For this review, use the dimensioned drawing (mm, ordinates from the lowest corner) and the shaded views. A direction names the side the tool comes from. Coordinates: 2 decimals unless noted, no trailing zeros. Loops run counter-clockwise (first coordinate to the right, second up) from the corner with the lowest first, then second, coordinate; pieces in that order, holes last. Notation, with made-up numbers: M 44.25,36.25 L 60.25,36.25 A23 ccw 60.25,64.25 Z; hole C 27.5,-7 d7. An arc over 180 degrees is marked long. Write item = value, one per line. Start each with the question number.
Q1. We need section B-B on x = 56. Give the boundary of the cut face in (y, z).
Q2. Wall thickness on probe 1 along X at (y, z) = (49.5, 6) (1 decimal); probe 2 along Y at (x, z) = (50, 29); probe 3 along X at (y, z) = (69, 44): over which ranges is each line inside the solid? List them lowest first.
Q3. We need section C-C on x = 30.5. Give the boundary of the cut face in (y, z) (1 decimal), and give its area (3 significant figures).
Q4. Mouldability with a two-part tool opening along Y and no side actions: class the marked faces 3, 4 and 5 as released by +Y, released by -Y, zero draft, split by the parting line, or undercut.
Q5. We need section A-A on z = 25. Give the boundary of the cut face in (x, y), and give its area (3 significant figures).
Q6. For the marked faces 1 and 2, list the 3-axis set-ups (+Z, -Z, +X, -X, +Y, -Y) from which the entire face can be reached by the end or side of a thin tool; tool diameter is ignored.
Q7. Clearance check with flat-ended pins moving along their axes: pin 1 Ø3 at (y, z) = (89.5, 21) entering from -X (1 decimal); pin 2 Ø2 at (x, z) = (86.5, 15) entering from -Y; pin 3 Ø4 at (x, y) = (217, 30.5) entering from +Z. State where each tip first meets the part, or that it passes through.
Q8. We need section D-D on z = 14. Give the boundary of the cut face in (x, y).
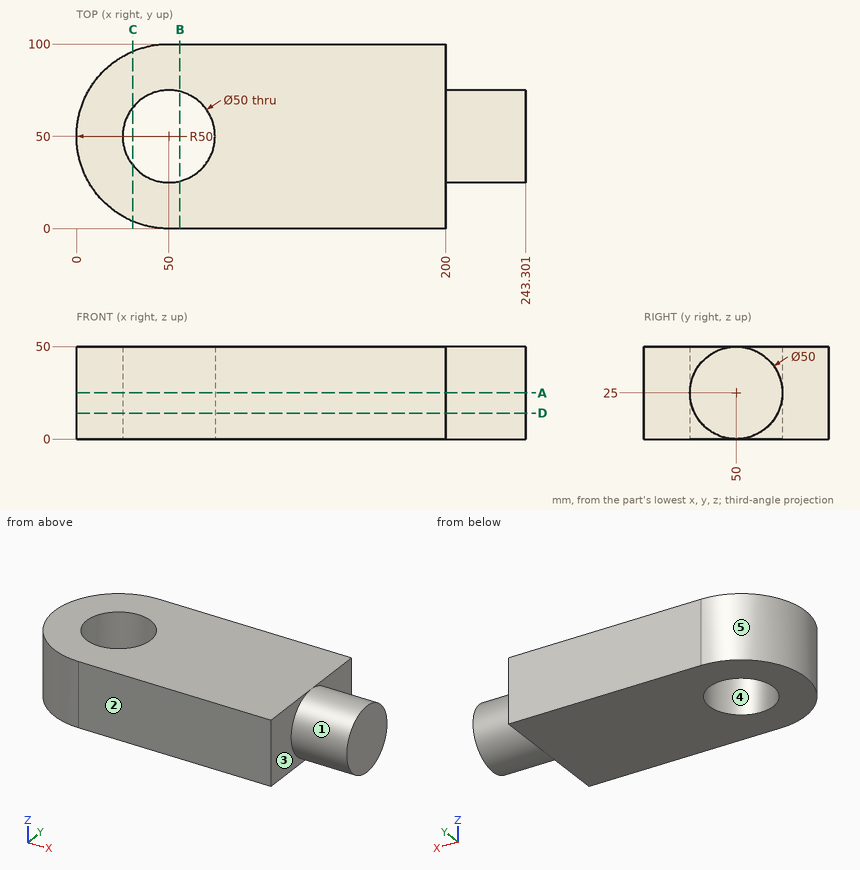
Returned:
q1.outline = M 0,0 L 25.73,0 L 25.73,50 L 0,50 Z; M 74.27,0 L 100,0 L 100,50 L 74.27,50 Z
q2.probe_1 = 0 to 25, 75 to 243.3
q2.probe_2 = 0 to 25, 75 to 100
q2.probe_3 = 3.75 to 33.75, 66.25 to 200
q3.outline = M 4,0 L 34.4,0 L 34.4,50 L 4,50 Z; M 65.6,0 L 96,0 L 96,50 L 65.6,50 Z
q3.area = 3,040 mm^2
q4.face_3 = zero draft
q4.face_4 = undercut
q4.face_5 = split by the parting line
q5.outline = M 50,0 L 200,0 L 200,25 L 243.3,25 L 243.3,75 L 200,75 L 200,100 L 50,100 A50 ccw Z; hole C 50,50 d50
q5.area = 19,100 mm^2
q6.face_1 = +X
q6.face_2 = +Z, -Z, +X, -X, -Y
q7.pin_1 = 17.5
q7.pin_2 = 0
q7.pin_3 = 42.85
q8.outline = M 50,0 L 200,0 L 200,27.55 L 243.3,27.55 L 243.3,72.45 L 200,72.45 L 200,100 L 50,100 A50 ccw Z; hole C 50,50 d50
